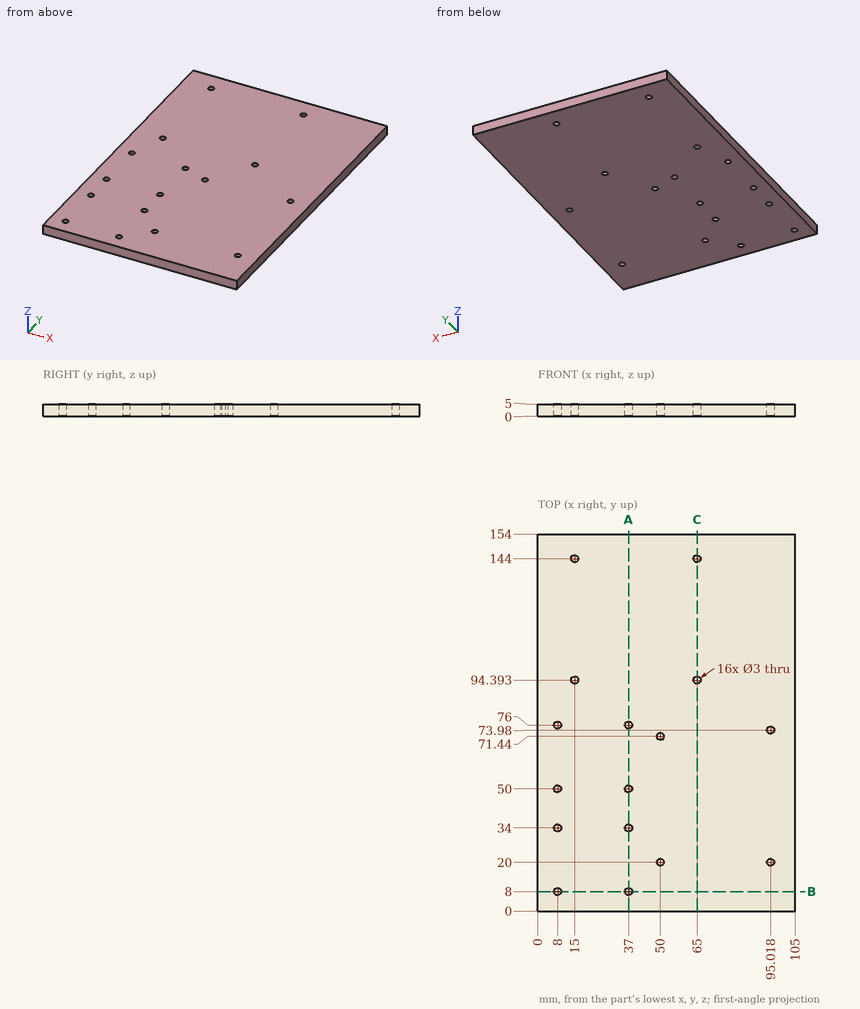
The drawing under review shows one solid part. Ordinate dimensions are in mm from its lowest x, y, z. Round coordinates to 2 decimals unless told otherwise and drop trailing zeros. Loops run counter-clockwise (first coordinate to the right, second up) from the corner with the lowest first, then second, coordinate; pieces in that order, holes last. Notation, with made-up numbers: (11.25, 74.25) - (31.25, 74.25) arc R13 ccw to (31.25, 87.25) - close; hole circle Ø4 at (51, 52.5). An arc over 180 degrees is marked (long way). One line per question, with ' | ' between items.
1. We need section A-A, the plane x = 37. State the section outline as (y, z) points, and give its area (3 significant figures).
Results are:
outline: (0, 0) - (6.5, 0) - (6.5, 5) - (0, 5) - close; (9.5, 0) - (32.5, 0) - (32.5, 5) - (9.5, 5) - close; (35.5, 0) - (48.5, 0) - (48.5, 5) - (35.5, 5) - close; (51.5, 0) - (74.5, 0) - (74.5, 5) - (51.5, 5) - close; (77.5, 0) - (154, 0) - (154, 5) - (77.5, 5) - close | area: 710 mm²
2. We need section B-B, the plane y = 8. State the section outline as (x, z) points.
Results are:
outline: (0, 0) - (6.5, 0) - (6.5, 5) - (0, 5) - close; (9.5, 0) - (35.5, 0) - (35.5, 5) - (9.5, 5) - close; (38.5, 0) - (105, 0) - (105, 5) - (38.5, 5) - close
3. For L1, parallel to X at y = 50, z = 3.6; L2, parallel to X at y = 20, z = 1.3; L3, parallel to Y at x = 37, z = 2.4, list the stretches that pass through material, from the lowest coordinate up. Write a range as [from, to].
Results are:
L1: x = [0, 6.5], [9.5, 35.5], [38.5, 105] | L2: x = [0, 48.5], [51.5, 93.52], [96.52, 105] | L3: y = [0, 6.5], [9.5, 32.5], [35.5, 48.5], [51.5, 74.5], [77.5, 154]
4. We need section C-C, the plane x = 65. State the section outline as (y, z) points.
Results are:
outline: (0, 0) - (92.89, 0) - (92.89, 5) - (0, 5) - close; (95.89, 0) - (142.5, 0) - (142.5, 5) - (95.89, 5) - close; (145.5, 0) - (154, 0) - (154, 5) - (145.5, 5) - close
5. Clearance check with a flat-ended pin moving along its axis: P1, Ø3.5, axis at x = 50, y = 20, coming from the -Z side. State where the tip first meets the part, or that it passes through.
Results are:
P1: stops at z = 0
